from build123d import *

# Parameters (mm, degrees)
SKETCH1_W           = 245
SKETCH1_H           = 118
BOSS_EXTRUDE1_DEPTH = 1.5
SKETCH2_W           = 37
SKETCH2_H           = 22
SKETCH2_W_2         = 60
SKETCH2_H_2         = 26
SKETCH2_W_3         = 45
SKETCH2_H_3         = 72
CUT_EXTRUDE1_DEPTH  = 2.5
SKETCH3_R           = 1.65
CUT_EXTRUDE2_DEPTH  = 10
FILLET1_R           = 4


with BuildPart() as part:
    # Sketch1 → Boss-Extrude1 (new body)
    with BuildSketch(Plane(origin=(0, 0, 0), x_dir=(1, 0, 0), z_dir=(0, 1, 0))):
        with Locations((122.5, 59)):
            Rectangle(SKETCH1_W, SKETCH1_H)
    extrude(amount=BOSS_EXTRUDE1_DEPTH)

    # Sketch2 → Cut-Extrude1 (cut, through all)
    with BuildSketch(Plane(origin=(0, 1.5, 0), x_dir=(1, 0, 0), z_dir=(0, 1, 0))):
        with Locations((18.5, 107)):
            Rectangle(SKETCH2_W, SKETCH2_H)
        with Locations((30, 13)):
            Rectangle(SKETCH2_W_2, SKETCH2_H_2)
        with Locations((226.5, 107)):
            Rectangle(SKETCH2_W, SKETCH2_H)
        with Locations((215, 13)):
            Rectangle(SKETCH2_W_2, SKETCH2_H_2)
        with Locations((122.5, 36)):
            Rectangle(SKETCH2_W_3, SKETCH2_H_3)
    extrude(amount=-CUT_EXTRUDE1_DEPTH, mode=Mode.SUBTRACT)

    # Sketch3 → Cut-Extrude2 (cut)
    with BuildSketch(Plane.XZ):
        with Locations((5, -31)):
            Circle(SKETCH3_R)
        with Locations((5, -91)):
            Circle(SKETCH3_R)
        with Locations((240, -31)):
            Circle(SKETCH3_R)
        with Locations((240, -91)):
            Circle(SKETCH3_R)
        with Locations((105, -77)):
            Circle(SKETCH3_R)
        with Locations((140, -77)):
            Circle(SKETCH3_R)
    extrude(amount=-CUT_EXTRUDE2_DEPTH, mode=Mode.SUBTRACT)

    # Fillet1
    fillet1_edges = [part.edges().sort_by_distance(p)[0] for p in [
        (0, 0.75, -26),
        (245, 0.75, -96),
        (245, 0.75, -26),
        (100, 0.75, 0),
        (145, 0.75, 0),
        (0, 0.75, -96),
    ]]
    fillet(fillet1_edges, radius=FILLET1_R)


solid = part.part
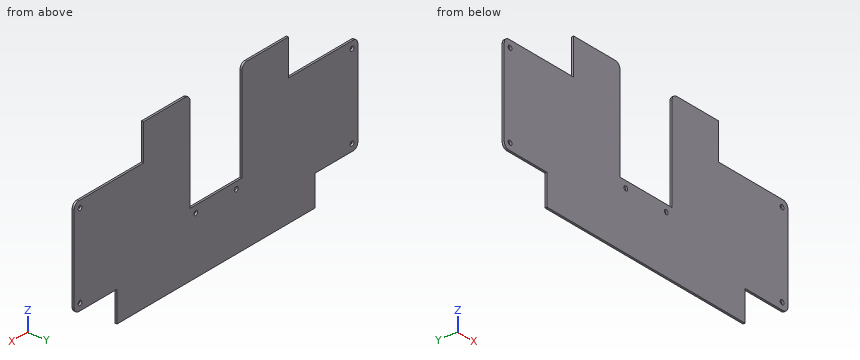
Geometry: final body of the model. Coordinates: model frame, mm. Coordinates: 2 decimals unless noted, no trailing zeros. Write each loop counter-clockwise with the first axis right and the second up, starting at its lowest first coordinate (ties: lowest second). Pieces come first, ordered by that corner, then holes. Notation, with made-up numbers: (-14.75, 41) - (3.25, 41) arc R19 cw to (3.25, 75) - close; hole circle Ø11 at (61.25, 36). An arc over 180 degrees is marked (long way). Return JSON: item names as keys, results as strings.
Item 1: Line query: L1, parallel to X at y = 0.4, z = -77; L2, parallel to X at y = 0.5, z = -91; L3, parallel to X at y = 0.5, z = -50. Output: solid intervals per line, ascending.
Completed:
{"L1": "x = 0 to 103.35, 106.65 to 138.35, 141.65 to 245", "L2": "x = 0 to 3.35, 6.65 to 238.35, 241.65 to 245", "L3": "x = 0 to 100, 145 to 245"}
Item 2: Section query A-A (z = -69). Output: boundary loops of the cut face in (x, y), and give its area (3 significant figures).
Completed:
{"outline": "(0, 0) - (100, 0) - (100, 1.5) - (0, 1.5) - close; (145, 0) - (245, 0) - (245, 1.5) - (145, 1.5) - close", "area": "300 mm2"}
Item 3: Section query D-D (x = 192.5). Output: boundary loops of the cut face in (y, z).
Completed:
{"outline": "(0, -118) - (1.5, -118) - (1.5, -26) - (0, -26) - close"}
Item 4: Pin query (flat end, axial travel): pin 1 Ø2.5 at (x, z) = (240, -31) entering from +Y; pin 2 Ø2 at (x, z) = (160, -40.5) entering from -Y; pin 3 Ø0.8 at (x, y) = (27, 0.5) entering from -Z. Return the tip coordinate at first contact, or that it passes through.
Completed:
{"pin 1": "passes through", "pin 2": "stops at y = 0", "pin 3": "stops at z = -96"}
Item 5: Section query C-C (x = 117.5). Output: boundary loops of the cut face in (y, z), and give its area (3 significant figures).
Completed:
{"outline": "(0, -118) - (1.5, -118) - (1.5, -72) - (0, -72) - close", "area": "69.0 mm2"}
Item 6: Section query B-B (y = 0.25). Output: boundary loops of the cut face in (x, z).
Completed:
{"outline": "(0, -92) arc R4 ccw to (4, -96) - (37, -96) - (37, -118) - (208, -118) - (208, -96) - (241, -96) arc R4 ccw to (245, -92) - (245, -30) arc R4 ccw to (241, -26) - (185, -26) - (185, 0) - (149, 0) arc R4 ccw to (145, -4) - (145, -72) - (100, -72) - (100, -4) arc R4 ccw to (96, 0) - (60, 0) - (60, -26) - (4, -26) arc R4 ccw to (0, -30) - close; hole circle Ø3.3 at (5, -91); hole circle Ø3.3 at (5, -31); hole circle Ø3.3 at (105, -77); hole circle Ø3.3 at (140, -77); hole circle Ø3.3 at (240, -91); hole circle Ø3.3 at (240, -31)"}
